Part model, mm, in its own coordinate system. Give positions to 0.01 mm unless a question says otherwise; leave off trailing zeros. Write each loop counter-clockwise with the first axis right and the second up, starting at its lowest first coordinate (ties: lowest second). Pieces come first, ordered by that corner, then holes. Notation, with made-up numbers: M 21,0 L 45,0 A11 cw 45,20 Z; hole C -19.5,9.25 d3. An arc over 180 degrees is marked long. Use a Markdown table: item, result. Add a question column.
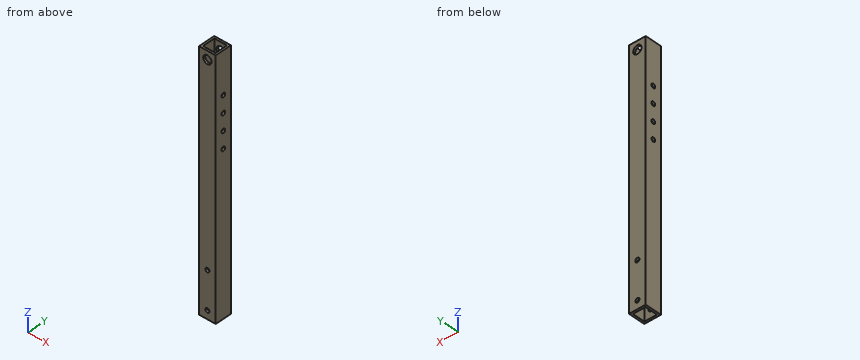
Autodesk Inventor part; units mm, degrees
ref_plane "YZ Plane" through (0, 0, 0) normal (1, 0, 0) x (0, 1, 0)
ref_plane "XZ Plane" through (0, 0, 0) normal (0, 1, 0) x (-1, 0, 0)
ref_plane "XY Plane" through (0, 0, 0) normal (0, 0, 1) x (1, 0, 0)
sketch "Sketch1" plane through (0, 0, 0) normal (0, 0, 1) x (1, 0, 0)
  line L0 (0, 0) -> (25.4, 0)
  line L1 (25.4, 0) -> (25.4, 25.4)
  line L2 (25.4, 25.4) -> (0, 25.4)
  line L3 (0, 25.4) -> (0, 0)
  line L4 (3.175, 3.175) -> (22.225, 3.175)
  line L5 (22.225, 3.175) -> (22.225, 22.225)
  line L6 (22.225, 22.225) -> (3.175, 22.225)
  line L7 (3.175, 22.225) -> (3.175, 3.175)
  dimension "d0" = 25.4
  dimension "d1" = 25.4
  dimension "d2" = 3.175
extrude "Extrusion1" add sketch "Sketch1" against normal blind 381
sketch "Sketch2" plane through (0, 25.4, 0) normal (0, 1, 0) x (1, 0, 0)
  line L0 (25.4, 381) -> (0, 381)
  line L1 (25.4, 0) -> (0, 0)
  line L2 (25.4, 0) -> (25.4, 381)
  point P0 (12.7, 368.3)
  point P1 (12.7, 311.15)
  point P2 (12.7, 12.7)
  dimension "d5" = 12.7
  dimension "d6" = 57.15
  dimension "d25" = 12.7
  dimension "d26" = 12.7
hole "Hole1" at (12.7, 25.4, -368.3) at (12.7, 25.4, -311.15) direction (0, -1, 0) diameter 6.35 depth 25.4 tip angle 118
sketch "Sketch3" plane through (25.4, 0, 0) normal (1, 0, 0) x (0, 0, -1)
  line L0 (0, 0) -> (0, 25.4)
  point P0 (63.5, 12.7)
  point P1 (0, 12.7)
  point P2 (88.9, 12.7)
  point P3 (114.3, 12.7)
  point P4 (0, 12.7)
  point P5 (139.7, 12.7)
  dimension "d14" = 63.5
  dimension "d15" = 25.4
  dimension "d16" = 25.4
  dimension "d24" = 139.7
hole "Hole2" at (25.4, 12.7, -63.5) at (25.4, 12.7, -88.9) at (25.4, 12.7, -114.3) at (25.4, 12.7, -139.7) direction (-1, 0, 0) diameter 6.35 depth 25.4 tip angle 118
hole "Hole3" at (12.7, 25.4, -12.7) direction (0, -1, 0) diameter 12.7 depth 25.4 tip angle 118
properties part number "bambar 12 in"
1. Flat gauge pin, fed straight in: pin 1 (5 mm diameter, centred on y = 12.7, z = -114.3, fed in from +X) (1 decimal). Where does the tip first touch, or does it go through?
2. Cut at A-A (z = -63.5). Write the cut outline in (x, y) (3 decimals).
3. Drill centre lines: probe 1 along Z at (x, y) = (24.6, 12.7) (3 decimals); probe 2 along Z at (x, y) = (12.7, 0.95) (3 decimals); probe 3 along X at (y, z) = (3.5, -76.5) (3 decimals). Where is each one in solid material? Low to high. Write a range as [from, to].
4. Cut at B-B (x = 12.7). Give the number of separate pieces and of enclosed holes in the cut face, then the cut area to 3 significant figures.
A:
| question | item | result |
|---|---|---|
| 1 | pin 1 | passes through |
| 2 | outline | M 0,0 L 25.4,0 L 25.4,9.525 L 22.225,9.525 L 22.225,3.175 L 3.175,3.175 L 3.175,9.525 L 0,9.525 Z; M 0,15.875 L 3.175,15.875 L 3.175,22.225 L 22.225,22.225 L 22.225,15.875 L 25.4,15.875 L 25.4,25.4 L 0,25.4 Z |
| 3 | probe 1 | z = [-381, -142.875], [-136.525, -117.475], [-111.125, -92.075], [-85.725, -66.675], [-60.325, 0] |
| 3 | probe 2 | z = [-381, -371.475], [-365.125, -314.325], [-307.975, -19.05], [-6.35, 0] |
| 3 | probe 3 | x = [0, 3.175], [22.225, 25.4] |
| 4 | separate pieces | 8 |
| 4 | enclosed holes | 0 |
| 4 | area | 2,260 mm² |
